Input: dimensioned drawing with shaded views. Units: mm. Origin: part minimum x, y, z. Coordinates: 2 decimals unless noted, no trailing zeros. Order: outer loops, then holes, each group sorted by start corner. A loop starts at its lowest first (then second) coordinate and runs counter-clockwise, first axis right, second up. Notation, with made-up numbers: (84.5, -12) -> (88.5, -12) arc R19 cw to (88.5, 12) -> close; hole circle Ø4 at (23.25, 2). An arc over 180 degrees is marked (long way). Answer in a Markdown table with one row per item. Add a question column.
1) Section query A-A on z = 18.5. Return the cut outline in (x, y), then the cut area to 3 significant figures.
2) Section query B-B on y = 117. Return the cut outline in (x, z).
3) Section query C-C on x = 33. Return the cut outline in (y, z), then the cut area to 3 significant figures.
4) Ray query, line 1 (Y direction, x = 8.5, z = 47.5); line 2 (X direction, y = 16.5, z = 39.5); line 3 (Z direction, x = 23.5, y = 107.5). Return the intervals inside material, ascending. Write a range as from..to.
5) Pull-direction query (Y, two-part tool) for the marked faces 1, 2 and 3; classes: +Y half, -Y half, draft (parallel to the pull), parting line (faces both ways), or undercut.
6) Contact query for flat-ended pins moving along their axis: P1, Ø12, axis at x = 27.5, y = 43, coming from the +Z side; P2, Ø2, axis at x = 35, z = 38, coming from the -Y side; P3, Ø2, axis at x = 40, z = 15.5, coming from the -Y side. Output: stop coordinate, or through.
7) Section query D-D on x = 43. Return the cut outline in (y, z), then the cut area to 3 significant figures.
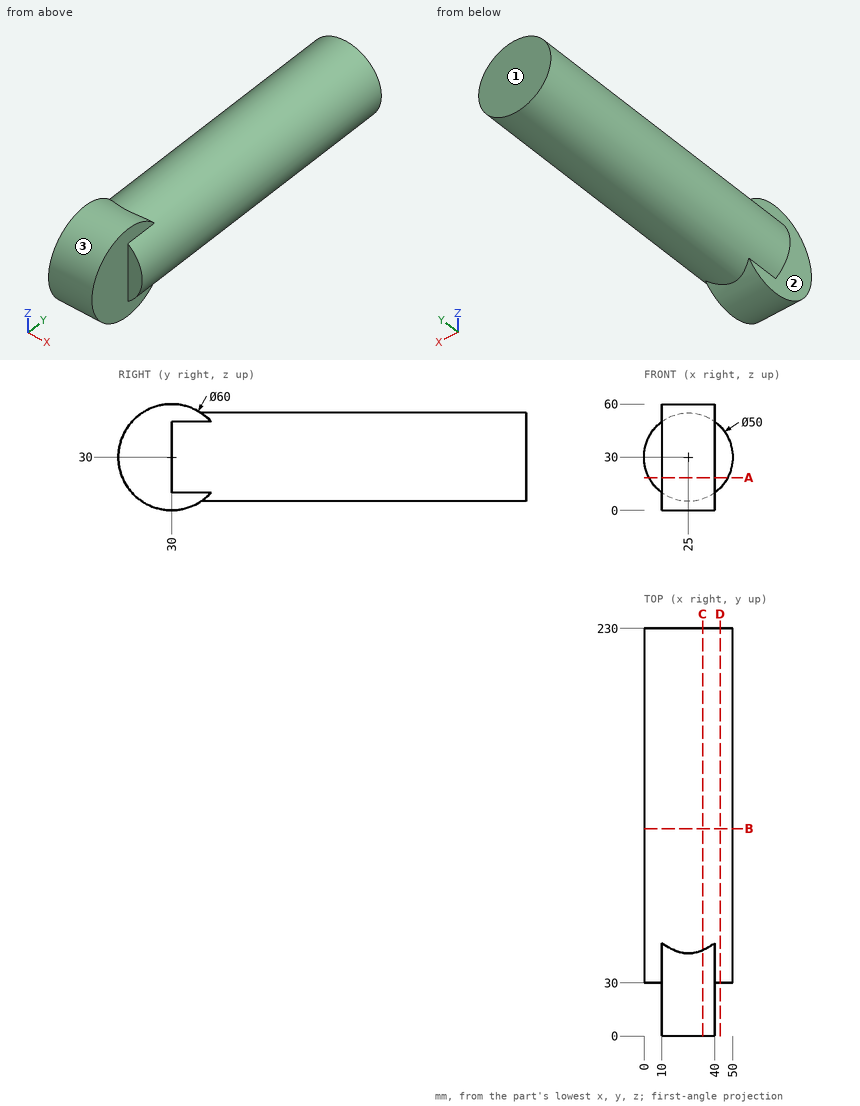
Result:
| question | item | result |
|---|---|---|
| 1 | outline | (2.8, 30) -> (10, 30) -> (10, 2.29) -> (40, 2.29) -> (40, 30) -> (47.2, 30) -> (47.2, 230) -> (2.8, 230) -> close |
| 1 | area | 9,710 mm2 |
| 2 | outline | circle Ø50 at (25, 30) |
| 3 | outline | (48.41, 6.31) -> (230, 6.31) -> (230, 53.69) -> (48.41, 53.69) arc R30 ccw (long way) to start |
| 3 | area | 11,000 mm2 |
| 4 | line 1 | 30..230 |
| 4 | line 2 | 10..40 |
| 4 | line 3 | 5.05..54.95 |
| 5 | face 1 | +Y half |
| 5 | face 2 | draft |
| 5 | face 3 | parting line |
| 6 | P1 | z = 59.17 |
| 6 | P2 | y = 0.83 |
| 6 | P3 | y = 3.21 |
| 7 | outline | (30, 12.65) -> (230, 12.65) -> (230, 47.35) -> (30, 47.35) -> close |
| 7 | area | 6,940 mm2 |
